Work out the finished part from the listing and answer in its coordinate system (mm). Give positions to 0.01 mm unless a question says otherwise; leave off trailing zeros. Loops run counter-clockwise (first coordinate to the right, second up) from the corner with the lowest first, then second, coordinate; pieces in that order, holes last. Notation, with made-up numbers: M -20,-24 L 6,-24 A21 ccw 6,0 Z; hole C 17.5,-18.75 d10. An arc over 180 degrees is marked long. Answer as a JSON object with one key per item and string values. Group by question number.
```python
from build123d import *

# Parameters (mm, degrees)
SKETCH_1_R      = 0.499999
SKETCH_1_R_2    = 0.3999992
SKETCH_1_R_3    = 0.7499985
SKETCH_1_W      = 15.49999948
SKETCH_1_H      = 15.49999948
EXTRUDE_1_DEPTH = 0.41148


with BuildPart() as part:
    # 草图1 → 凸台-拉伸1 (new body)
    with BuildSketch(Plane.XY):
        Polygon((1.5257399, 2.2389465), (1.6265017, 1.99568562), (1.78679094, 1.78679094), (1.99568562, 1.6265017), (2.2389465, 1.5257399), (2.50000008, 1.49137116), (38.4999992, 1.49999954), (38.4999992, 1.49137116), (38.76105278, 1.5257399), (39.00431366, 1.6265017), (39.21320834, 1.78679094), (39.37349758, 1.99568562), (39.47425938, 2.2389465), (39.50862812, 2.50000008), (39.49999974, 28.49999888), (39.50862812, 28.49999888), (39.47425938, 28.76105246), (39.37349758, 29.00431334), (39.21320834, 29.21320802), (39.00431366, 29.37349726), (38.76105278, 29.47425906), (38.4999992, 29.5086278), (2.50000008, 29.49999942), (2.50000008, 29.5086278), (2.2389465, 29.47425906), (1.99568562, 29.37349726), (1.78679094, 29.21320802), (1.6265017, 29.00431334), (1.5257399, 28.76105246), (1.49137116, 28.49999888), (1.49999954, 2.50000008), (1.49137116, 2.50000008), align=None)
        with Locations(Location((38.0000002, 27.99999988, 0), (0, 0, 180))):
            Circle(SKETCH_1_R, mode=Mode.SUBTRACT)
        with Locations(Location((33.77000104, 27.50000088, 0), (0, 0, 180))):
            Circle(SKETCH_1_R, mode=Mode.SUBTRACT)
        with Locations(Location((31.23000104, 27.50000088, 0), (0, 0, 180))):
            Circle(SKETCH_1_R, mode=Mode.SUBTRACT)
        with Locations(Location((19.0000001, 25.4999998, 0), (0, 0, 180))):
            Circle(SKETCH_1_R_2, mode=Mode.SUBTRACT)
        with Locations(Location((16.99999902, 25.4999998, 0), (0, 0, 180))):
            Circle(SKETCH_1_R_2, mode=Mode.SUBTRACT)
        with Locations(Location((21.00000118, 25.4999998, 0), (0, 0, 180))):
            Circle(SKETCH_1_R_2, mode=Mode.SUBTRACT)
        with Locations(Location((34.00000058, 7.00000124, 0), (0, 0, 180))):
            Circle(SKETCH_1_R, mode=Mode.SUBTRACT)
        with Locations(Location((34.00000058, 24.00000026, 0), (0, 0, 180))):
            Circle(SKETCH_1_R, mode=Mode.SUBTRACT)
        with Locations(Location((38.0000002, 2.99999908, 0), (0, 0, 180))):
            Circle(SKETCH_1_R, mode=Mode.SUBTRACT)
        with Locations(Location((31.5000005, 16.76999948, 0), (0, 0, 180))):
            Circle(SKETCH_1_R, mode=Mode.SUBTRACT)
        with Locations(Location((27.29999874, 25.4999998, 0), (0, 0, 180))):
            Circle(SKETCH_1_R_3, mode=Mode.SUBTRACT)
        with Locations(Location((31.5000005, 14.22999948, 0), (0, 0, 180))):
            Circle(SKETCH_1_R, mode=Mode.SUBTRACT)
        with Locations(Location((14.70000108, 25.4999998, 0), (0, 0, 180))):
            Circle(SKETCH_1_R_3, mode=Mode.SUBTRACT)
        with Locations(Location((12.0000014, 25.0000008, 0), (0, 0, 180))):
            Circle(SKETCH_1_R_2, mode=Mode.SUBTRACT)
        with Locations(Location((10.00000032, 25.0000008, 0), (0, 0, 180))):
            Circle(SKETCH_1_R_2, mode=Mode.SUBTRACT)
        with Locations(Location((6.9999987, 24.00000026, 0), (0, 0, 180))):
            Circle(SKETCH_1_R, mode=Mode.SUBTRACT)
        with Locations(Location((2.99999908, 27.99999988, 0), (0, 0, 180))):
            Circle(SKETCH_1_R, mode=Mode.SUBTRACT)
        with Locations(Location((8.99999978, 17.54000048, 0), (0, 0, 180))):
            Circle(SKETCH_1_R, mode=Mode.SUBTRACT)
        with Locations(Location((8.99999978, 15.00000048, 0), (0, 0, 180))):
            Circle(SKETCH_1_R, mode=Mode.SUBTRACT)
        with Locations(Location((8.99999978, 12.46000048, 0), (0, 0, 180))):
            Circle(SKETCH_1_R, mode=Mode.SUBTRACT)
        with Locations(Location((6.9999987, 7.00000124, 0), (0, 0, 180))):
            Circle(SKETCH_1_R, mode=Mode.SUBTRACT)
        with Locations(Location((2.99999908, 2.99999908, 0), (0, 0, 180))):
            Circle(SKETCH_1_R, mode=Mode.SUBTRACT)
        with Locations((20.49999964, 15.49999948)):
            Rectangle(SKETCH_1_W, SKETCH_1_H, mode=Mode.SUBTRACT)
    extrude(amount=-EXTRUDE_1_DEPTH)


solid = part.part
```
Item 1: For a pull along Y with two mould halves and no side action, classify faces 1 (the flat face through (29, 16, 0)), 2 (the cylindrical face through (34.27, 27.48, -0.2)) as pulls with the +Y half, pulls with the -Y half, needs draft (parallel to the pull), parting line crosses it, or undercut.
Item 2: A cutting plane is placed at A-A (y = 3). Determine the outline of the cut face in (x, z).
Item 3: A cutting plane is placed at D-D (z = -0.1). Give the number of separate pieces and of enclosed holes in the cut face, and give its area (3 significant figures).
Item 4: Find the intervals of material crossed by probe 1 along Y at (x, z) = (9, -0.05); probe 2 along X at (y, z) = (3, -0.2); probe 3 along X at (y, z) = (25.5, -0.2), in increasing order. Write a range as [from, to].
Item 5: A cutting plane is placed at C-C (x = 25.5). Determine the outline of the cut face in (y, z), and give its area (3 significant figures).
Item 6: A cutting plane is placed at B-B (x = 9). Determine the outline of the cut face in (y, z), and give its area (3 significant figures).
Item 7: Given pin 1 Ø10 at (x, y) = (17, 22.5) entering from +Z; pin 2 Ø6 at (x, y) = (19.5, 12.5) entering from +Z, each flat-ended and moving along its own axis, determine where each tip first touches the part or whether it passes through.
The answers:
{
 "1": {"face 1": "needs draft", "face 2": "undercut"},
 "2": {"outline": "M 1.5,-0.41 L 2.5,-0.41 L 2.5,0 L 1.5,0 Z; M 3.5,-0.41 L 37.5,-0.41 L 37.5,0 L 3.5,0 Z; M 38.5,-0.41 L 39.51,-0.41 L 39.51,0 L 38.5,0 Z"},
 "3": {"separate pieces": "1", "enclosed holes": "23", "area": "806 mm^2"},
 "4": {"probe 1": "y = [1.49, 11.96], [12.96, 14.5], [15.5, 17.04], [18.04, 29.5]", "probe 2": "x = [1.5, 2.5], [3.5, 37.5], [38.5, 39.51]", "probe 3": "x = [1.49, 13.95], [15.45, 16.6], [17.4, 18.6], [19.4, 20.6], [21.4, 26.55], [28.05, 39.5]"},
 "5": {"outline": "M 1.5,-0.41 L 7.75,-0.41 L 7.75,0 L 1.5,0 Z; M 23.25,-0.41 L 29.51,-0.41 L 29.51,0 L 23.25,0 Z", "area": "5.15 mm^2"},
 "6": {"outline": "M 1.49,-0.41 L 11.96,-0.41 L 11.96,0 L 1.49,0 Z; M 12.96,-0.41 L 14.5,-0.41 L 14.5,0 L 12.96,0 Z; M 15.5,-0.41 L 17.04,-0.41 L 17.04,0 L 15.5,0 Z; M 18.04,-0.41 L 29.5,-0.41 L 29.5,0 L 18.04,0 Z", "area": "10.3 mm^2"},
 "7": {"pin 1": "stops at z = 0", "pin 2": "passes through"}
}
